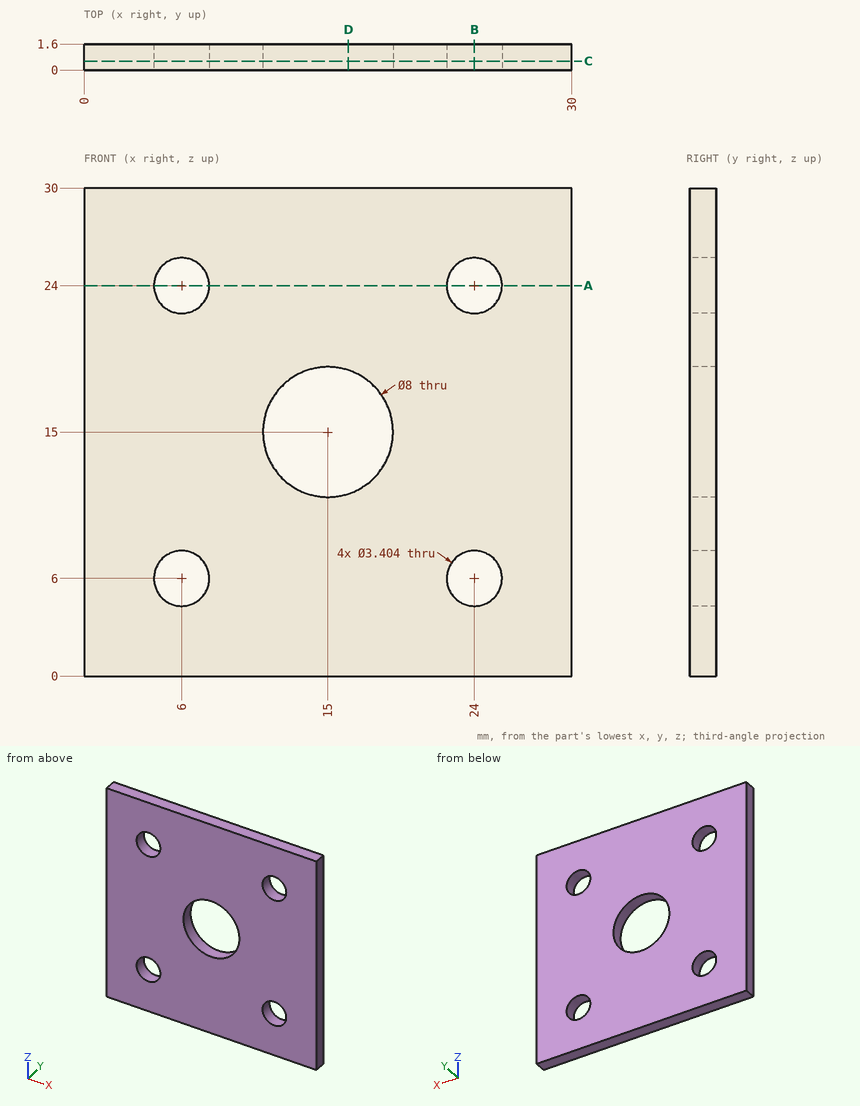
Can you work these out from the drawing? Everything is in mm from the part's minimum corner. Coordinates: 2 decimals unless noted, no trailing zeros. Order: outer loops, then holes, each group sorted by start corner. A loop starts at its lowest first (then second) coordinate and runs counter-clockwise, first axis right, second up. Notation, with made-up numbers: (42.5, 9) -> (85.5, 9) arc R31 cw to (85.5, 42) -> close; hole circle Ø6 at (-32.75, 77). An arc over 180 degrees is marked (long way). Return JSON: item names as keys, results as strings.
1) If we section it at D-D on x = 16.25: List the corners of the cut face in (y, z) for me.
Conclusion:
{"outline": "(0, 0) -> (1.6, 0) -> (1.6, 11.2) -> (0, 11.2) -> close; (0, 18.8) -> (1.6, 18.8) -> (1.6, 30) -> (0, 30) -> close"}
2) I'm going to push a flat-ended pin straight in: P1, Ø5, axis at x = 15, z = 15, coming from the +Y side. Where does the tip first touch, or does it pass through?
Conclusion:
{"P1": "passes through"}
3) If I drill on probe 1 along X at (y, z) = (0.5, 24); probe 2 along Z at (x, y) = (24.5, 0.5), over which ranges is the centre line in solid material (lowest first)?
Conclusion:
{"probe 1": "x = 0 to 4.3, 7.7 to 22.3, 25.7 to 30", "probe 2": "z = 0 to 4.37, 7.63 to 22.37, 25.63 to 30"}
4) If we section it at A-A on z = 24: List the corners of the cut face in (x, y) for me.
Conclusion:
{"outline": "(0, 0) -> (4.3, 0) -> (4.3, 1.6) -> (0, 1.6) -> close; (7.7, 0) -> (22.3, 0) -> (22.3, 1.6) -> (7.7, 1.6) -> close; (25.7, 0) -> (30, 0) -> (30, 1.6) -> (25.7, 1.6) -> close"}
5) If we section it at C-C on y = 0.55: List the corners of the cut face in (x, z) for me, plus the area to 3 significant figures.
Conclusion:
{"outline": "(0, 0) -> (30, 0) -> (30, 30) -> (0, 30) -> close; hole circle Ø3.4 at (6, 6); hole circle Ø3.4 at (6, 24); hole circle Ø8 at (15, 15); hole circle Ø3.4 at (24, 6); hole circle Ø3.4 at (24, 24)", "area": "813 mm²"}
6) If we section it at B-B on x = 24: List the corners of the cut face in (y, z) for me.
Conclusion:
{"outline": "(0, 0) -> (1.6, 0) -> (1.6, 4.3) -> (0, 4.3) -> close; (0, 7.7) -> (1.6, 7.7) -> (1.6, 22.3) -> (0, 22.3) -> close; (0, 25.7) -> (1.6, 25.7) -> (1.6, 30) -> (0, 30) -> close"}
